Autodesk Inventor part; units mm, degrees
ref_plane "YZ Plane" through (0, 0, 0) normal (1, 0, 0) x (0, 1, 0)
ref_plane "XZ Plane" through (0, 0, 0) normal (0, 1, 0) x (-1, 0, 0)
ref_plane "XY Plane" through (0, 0, 0) normal (0, 0, 1) x (1, 0, 0)
sketch "Sketch1" plane through (0, 0, 0) normal (0, 1, 0) x (-1, 0, 0)
  circle A0 centre (0, 0) radius 1.7
  arc A1 (-3.175, 0) -> (3.175, 0) centre (0, 0) ccw
  line L0 (-3.175, 0) -> (-3.175, 7.239)
  line L1 (3.175, 7.239) -> (3.175, 0)
  arc A2 (3.175, 7.239) -> (-3.175, 7.239) centre (0, 7.239) ccw
  dimension "d0" = 3.4
  dimension "d1" = 6.35
  dimension "d6" = 6.35
  dimension "d8" = 7.239
extrude "Extrusion1" add sketch "Sketch1" along normal blind 5.9944
properties part number "Limit switch trigger spacer"
Could you check a few things on this model? Use its own coordinates, in mm. Coordinates: 2 decimals unless noted, no trailing zeros. Write each loop counter-clockwise with the first axis right and the second up, starting at its lowest first coordinate (ties: lowest second). Pieces come first, ordered by that corner, then holes. Notation, with made-up numbers: (42.5, 35) -> (49.5, 35) arc R22 cw to (49.5, 69) -> close; hole circle Ø6 at (19, 40). An arc over 180 degrees is marked (long way). Write item = value, one per line. Start each with the question number.
(1) I want a section at A-A (x = 0). Please give me the cut outline in (y, z) (3 decimals), plus the area to 3 significant figures.
(2) We'd pull the mould along X, two halves only. Please class faces 1 (the face through (-3.175, 3, 4)), 2 (the face through (0, 5.994, 4)), 3 (the face through (0.37, 2.96, 1.66)): released by +X, released by -X, zero draft, split by the parting line, or undercut.
(3) I want a section at B-B (z = -0.5). Please give me the cut outline in (x, y), plus the area to 3 significant figures.
(4) I want a section at D-D (x = -2). Please give me the cut outline in (y, z).
(5) I want a section at C-C (y = 4.2). Please give me the cut outline in (x, z) (3 decimals), plus the area to 3 significant figures.
(6) Will these pins go through, and if not, where does the flat tip stop? pin 1 (2 mm diameter, centred on x = 2, y = 4.5, fed in from -Z); pin 2 (2.5 mm diameter, centred on x = 0, z = 0, fed in from -Y).
(7) I need wall thicknesses on line 1 (Z direction, x = 0, y = 2.6) (3 decimals); line 2 (X direction, y = 5.65, z = -1.25); line 3 (Z direction, x = -0.75, y = 4.5). Which ranges of each line are inside material? Lowest first, please. Write a range as [from, to].
Result set:
q1.outline = (0, -3.175) -> (5.994, -3.175) -> (5.994, -1.7) -> (0, -1.7) -> close; (0, 1.7) -> (5.994, 1.7) -> (5.994, 10.414) -> (0, 10.414) -> close
q1.area = 61.1 mm2
q2.face_1 = released by -X
q2.face_2 = zero draft
q2.face_3 = undercut
q3.outline = (-3.14, 0) -> (-1.62, 0) -> (-1.62, 5.99) -> (-3.14, 5.99) -> close; (1.62, 0) -> (3.14, 0) -> (3.14, 5.99) -> (1.62, 5.99) -> close
q3.area = 18.1 mm2
q4.outline = (0, -2.47) -> (5.99, -2.47) -> (5.99, 9.7) -> (0, 9.7) -> close
q5.outline = (-3.175, 0) arc R3.175 ccw to (3.175, 0) -> (3.175, 7.239) arc R3.175 ccw to (-3.175, 7.239) -> close; hole circle Ø3.4 at (0, 0)
q5.area = 68.6 mm2
q6.pin_1 = -3.01
q6.pin_2 = through
q7.line_1 = [-3.175, -1.7], [1.7, 10.414]
q7.line_2 = [-2.92, -1.15], [1.15, 2.92]
q7.line_3 = [-3.09, -1.53], [1.53, 10.32]
